Part model, mm, in its own coordinate system. A direction names the side the tool comes from. Give positions to 0.01 mm unless a question says otherwise; leave off trailing zeros. Write each loop counter-clockwise with the first axis right and the second up, starting at its lowest first coordinate (ties: lowest second). Pieces come first, ordered by that corner, then holes. Notation, with made-up numbers: (0, -2) - (31, -2) arc R16 cw to (31, 15) - close; hole circle Ø4 at (76, -36). An arc over 180 degrees is marked (long way). Answer as a JSON object with one key per item and string values. Group by question number.
```python
from build123d import *

# Parameters (mm, degrees)
SKETCH1_R           = 1.6
BOSS_EXTRUDE1_DEPTH = 1.57
SKETCH2_W           = 4.53
SKETCH2_H           = 2.42
BOSS_EXTRUDE2_DEPTH = 2
SKETCH3_W           = 15.24
SKETCH3_H           = 2.54
BOSS_EXTRUDE3_DEPTH = 10


with BuildPart() as part:
    # Sketch1 → Boss-Extrude1 (new body)
    with BuildSketch(Plane(origin=(0, 0, 0), x_dir=(1, 0, 0), z_dir=(0, 1, 0))):
        with BuildLine():
            Line((-7.76, -6.25), (7.76, -6.25))
            Line((7.76, -6.25), (7.76, -2.41))
            Line((7.76, -2.41), (10, -2.41))
            ThreePointArc((10, -2.41), (12.41, 0), (10, 2.41))
            Line((10, 2.41), (7.76, 2.41))
            Line((7.76, 2.41), (7.76, 6.25))
            Line((7.76, 6.25), (-7.76, 6.25))
            Line((-7.76, 6.25), (-7.76, 2.41))
            Line((-7.76, 2.41), (-10, 2.41))
            ThreePointArc((-10, 2.41), (-12.41, 0), (-10, -2.41))
            Line((-10, -2.41), (-7.76, -2.41))
            Line((-7.76, -2.41), (-7.76, -6.25))
        make_face()
        with Locations(Location((-10, 0, 0), (0, 0, 270))):
            Circle(SKETCH1_R, mode=Mode.SUBTRACT)
        with Locations(Location((10, 0, 0), (0, 0, 270))):
            Circle(SKETCH1_R, mode=Mode.SUBTRACT)
    extrude(amount=BOSS_EXTRUDE1_DEPTH)

    # Sketch2 → Boss-Extrude2 (add)
    with BuildSketch(Plane(origin=(0, 1.57, 0), x_dir=(1, 0, 0), z_dir=(0, 1, 0))):
        with Locations((0, -2.1)):
            Rectangle(SKETCH2_W, SKETCH2_H)
    extrude(amount=BOSS_EXTRUDE2_DEPTH)

    # Sketch3 → Boss-Extrude3 (add)
    with BuildSketch(Plane.XZ):
        with Locations((0, -4.88)):
            Rectangle(SKETCH3_W, SKETCH3_H)
    extrude(amount=BOSS_EXTRUDE3_DEPTH)


solid = part.part
```
1) Drop flat-ended pins along their axis: P1, Ø1.6, axis at x = -1, y = 2.5, coming from the -Z side; P2, Ø1.9, axis at x = -10, z = 0, coming from the -Y side; P3, Ø3, axis at x = -1, y = -6.5, coming from the +Z side; P4, Ø5, axis at x = 3.5, y = -6, coming from the -Z side. Give the stop position or say it passes through.
2) Band-saw the part on D-D (z = -5.5). List the corners of the cut face in (x, y).
3) Band-saw the part on C-C (x = -10.25). List the corners of the cut face in (y, z).
4) Probe line 1 (X direction, y = 0.8, z = 0); line 2 (Z direction, x = -1, y = -2.5); line 3 (Y direction, x = 0.5, z = -4.75). List the from-to ranges inside material, lowest first.
5) Which spindle directions (+Z, -Z, +X, -X, +Y, -Y) get a long thin tool onto all of the face, cutting with end or side? Do faces 1 (the flat face through (0, -5, -3.61)), 2 (the flat face through (2.265, 3, 2)), 3 (the flat face through (0, 3, 0.89)), 4 (the flat face through (7.76, 1, -4)). Say none if no direction does.
6) Band-saw the part on B-B (x = -2). List the corners of the cut face in (y, z), plus the area to 3 significant figures.
7) Band-saw the part on A-A (z = 0). List the corners of the cut face in (x, y).
8) Mould opens along X. For faces 5 (the flat face through (-2.265, 3, 2)), 6 (the cylindrical face through (8.44, 0.77, -0.35)), 7 (the flat face through (0, 1, -6.25)) say: pulls with the +X half, pulls with the -X half, needs draft (parallel to the pull), parting line crosses it, or undercut.
Verdict:
{
 "1": {"P1": "z = 0.89", "P2": "through", "P3": "z = -3.61", "P4": "z = -6.15"},
 "2": {"outline": "(-7.76, 0) - (-7.62, 0) - (-7.62, -10) - (7.62, -10) - (7.62, 0) - (7.76, 0) - (7.76, 1.57) - (-7.76, 1.57) - close"},
 "3": {"outline": "(0, -2.4) - (1.57, -2.4) - (1.57, -1.58) - (0, -1.58) - close; (0, 1.58) - (1.57, 1.58) - (1.57, 2.4) - (0, 2.4) - close"},
 "4": {"line 1": "-12.41 to -11.6, -8.4 to 8.4, 11.6 to 12.41", "line 2": "-6.15 to -3.61", "line 3": "-10 to 1.57"},
 "5": {"face 1": "+Z, +X, -X, -Y", "face 2": "+Z, -Z, +X, +Y", "face 3": "-Z, +X, -X, +Y", "face 4": "-Z, +X, +Y, -Y"},
 "6": {"outline": "(-10, -6.15) - (0, -6.15) - (0, -6.25) - (1.57, -6.25) - (1.57, 0.89) - (3.57, 0.89) - (3.57, 3.31) - (1.57, 3.31) - (1.57, 6.25) - (0, 6.25) - (0, -3.61) - (-10, -3.61) - close", "area": "49.9 mm2"},
 "7": {"outline": "(-12.41, 0) - (-11.6, 0) - (-11.6, 1.57) - (-12.41, 1.57) - close; (-8.4, 0) - (8.4, 0) - (8.4, 1.57) - (-8.4, 1.57) - close; (11.6, 0) - (12.41, 0) - (12.41, 1.57) - (11.6, 1.57) - close"},
 "8": {"face 5": "pulls with the -X half", "face 6": "undercut", "face 7": "needs draft"}
}
